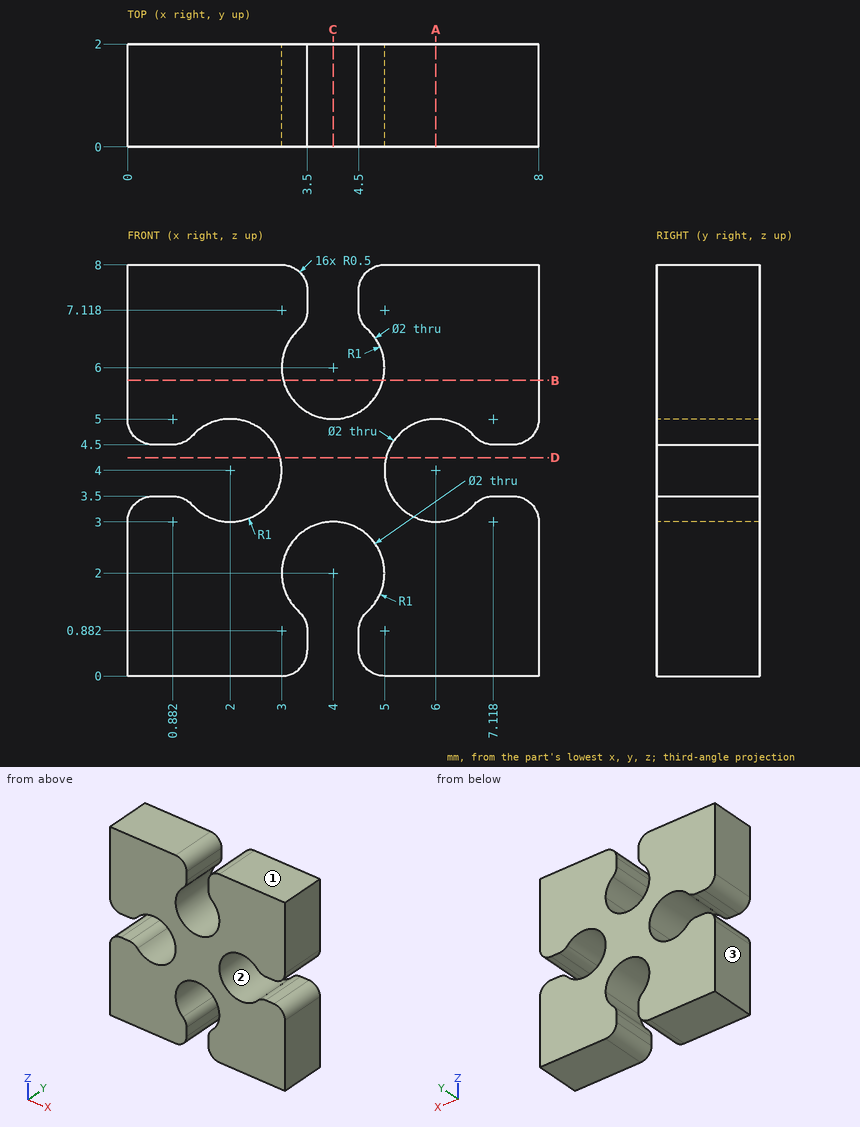
Study the drawing (mm; zero at the part's minimum x, y, z) and answer. Coordinates: 2 decimals unless noted, no trailing zeros. Order: outer loops, then holes, each group sorted by start corner. A loop starts at its lowest first (then second) coordinate and runs counter-clockwise, first axis right, second up. Notation, with made-up numbers: M 81.25,37 L 86.25,37 A10 ccw 86.25,46 Z; hole C 71,15 d9. An arc over 180 degrees is marked long. Answer as a JSON object with one key per item and string values. Group by question number.
1. Straight lines are drawn through the part: line 1 (Z direction, x = 6, y = 1.1); line 2 (X direction, y = 1.75, z = 7.25). For each, find the intervals that lie inside material, in ascending order.
2. Section B-B on z = 5.75 is taken. Write down the section's boundary in (x, y), then the cut area to 3 significant figures.
3. Section C-C on x = 4 is taken. Write down the section's boundary in (y, z).
4. A flat-ended cylindrical pin translates along its axis: P1, Ø2.5, axis at x = 6, z = 4, coming from the +Y side. Find the tip coordinate at first contact, or state that the pin passes through.
5. Determine the mould class of the marked faces 1, 2 and 3 for opening direction Z: released by +Z, released by -Z, zero draft, split by the parting line, or undercut.
6. Section D-D on z = 4.25 is taken. Write down the section's boundary in (x, y), then the cut area to 3 significant figures.
7. Section A-A on x = 6 is taken. Write down the section's boundary in (y, z).
Values follow:
{
 "1": {"line 1": "0 to 3, 5 to 8", "line 2": "0 to 3.5, 4.5 to 8"},
 "2": {"outline": "M 0,0 L 3.03,0 L 3.03,2 L 0,2 Z; M 4.97,0 L 8,0 L 8,2 L 4.97,2 Z", "area": "12.1 mm2"},
 "3": {"outline": "M 0,3 L 2,3 L 2,5 L 0,5 Z"},
 "4": {"P1": "y = 2"},
 "5": {"face 1": "released by +Z", "face 2": "undercut", "face 3": "zero draft"},
 "6": {"outline": "M 2.97,0 L 5.03,0 L 5.03,2 L 2.97,2 Z", "area": "4.13 mm2"},
 "7": {"outline": "M 0,0 L 2,0 L 2,3 L 0,3 Z; M 0,5 L 2,5 L 2,8 L 0,8 Z"}
}
